from build123d import *

# Parameters (mm, degrees)
SKETCH1_W           = 31
SKETCH1_H           = 12
BOSS_EXTRUDE1_DEPTH = 11.3
SKETCH3_W           = 2
SKETCH3_H           = 4.45
BOSS_EXTRUDE2_DEPTH = 12
SKETCH4_W           = 2
SKETCH4_H           = 4.45
BOSS_EXTRUDE3_DEPTH = 12
SKETCH5_R           = 1
CUT_EXTRUDE1_DEPTH  = 36.285443174
SKETCH6_R           = 6
BOSS_EXTRUDE4_DEPTH = 3
SKETCH8_R           = 4
BOSS_EXTRUDE5_DEPTH = 3


with BuildPart() as part:
    # Sketch1 → Boss-Extrude1 (new, symmetric)
    with BuildSketch(Plane(origin=(0, 0, 0), x_dir=(1, 0, 0), z_dir=(0, 1, 0))):
        Rectangle(SKETCH1_W, SKETCH1_H)
    extrude(amount=BOSS_EXTRUDE1_DEPTH, both=True)

    # Sketch3 → Boss-Extrude2 (add)
    with BuildSketch(Plane(origin=(0, 0, -6), x_dir=(-1, 0, 0), z_dir=(0, 0, -1))):
        with Locations((14.5, 13.525)):
            Rectangle(SKETCH3_W, SKETCH3_H)
    extrude(amount=-BOSS_EXTRUDE2_DEPTH)

    # Sketch4 → Boss-Extrude3 (add)
    with BuildSketch(Plane(origin=(0, 0, -6), x_dir=(-1, 0, 0), z_dir=(0, 0, -1))):
        with Locations((14.5, -13.525)):
            Rectangle(SKETCH4_W, SKETCH4_H)
    extrude(amount=-BOSS_EXTRUDE3_DEPTH)

    # Sketch5 → Cut-Extrude1 (cut, through all)
    with BuildSketch(Plane.ZY.offset(15.5)):
        with Locations((0, 14.65)):
            Circle(SKETCH5_R)
        with Locations((0, -14.65)):
            Circle(SKETCH5_R)
    extrude(amount=-CUT_EXTRUDE1_DEPTH, mode=Mode.SUBTRACT)

    # Sketch6 → Boss-Extrude4 (add, symmetric)
    with BuildSketch(Plane.ZY.offset(15.5)):
        with Locations((0, 6.07521459)):
            Circle(SKETCH6_R)
    extrude(amount=BOSS_EXTRUDE4_DEPTH, both=True)

    # Sketch8 → Boss-Extrude5 (add, symmetric)
    with BuildSketch(Plane.ZY.offset(18.5)):
        with Locations((0, 6.07521459)):
            Circle(SKETCH8_R)
    extrude(amount=BOSS_EXTRUDE5_DEPTH, both=True)


solid = part.part
Check sheet for the modelled part. Datum: model origin and axes. Units: mm. A direction names the side the tool comes from. Round coordinates to 2 decimals unless told otherwise and drop trailing zeros. Loops run counter-clockwise (first coordinate to the right, second up) from the corner with the lowest first, then second, coordinate; pieces in that order, holes last.
1. Sectioned sample at A-A on y = 14.65. Record the boundary of the cut face in (x, z), and give its area (3 significant figures).
2. Sectioned sample at C-C on x = -13. Record the boundary of the cut face in (y, z), and give its area (3 significant figures).
3. Mould release check, pull along Z, two halves, no side actions. Record for faces 1 (the cylindrical face through (-14.51, 15.49, 0.54)), 2 (the flat face through (-18.5, 2, 1)), 3 (the cylindrical face through (-13.007, 12.075, 0.043)): released by +Z, released by -Z, zero draft, split by the parting line, or undercut.
4. Sectioned sample at D-D on y = -0.5. Record the boundary of the cut face in (x, z), and give its area (3 significant figures).
5. Scan lines: probe 1 along Y at (x, z) = (-14, -0.5); probe 2 along Y at (x, z) = (4.5, -3.75); probe 3 along X at (y, z) = (-10, -3). Record each from-to range of solid material in increasing order.
6. Gauge pin test, flat ends, axial feed: pin 1 Ø1.2 at (y, z) = (14.65, 0) entering from +X; pin 2 Ø6 at (y, z) = (-6.5, -4.5) entering from -X; pin 3 Ø2 at (y, z) = (14.5, -0.5) entering from +X; pin 4 Ø0.9 at (y, z) = (12, -1) entering from +X. Record the tip position at first contact, or that the pin passes through.
7. Set-up check for faces 4 (the cylindrical face through (-20.02, 10.04, -0.52)), 5 (the flat face through (0, 0, -6)), 6 (the cylindrical face through (-14.514, -14.35, 0.954)), 7 (the flat face through (1, -11.3, 0)), 8 (the flat face through (-15.5, 13, 0)): record each of +Z, -Z, +X, -X, +Y, -Y from which the full face is reachable in a straight line by a thin tool's end or side.
8. Sectioned sample at B-B on z = 0. Record the boundary of the cut face in (x, y), and give its area (3 significant figures).
Recorded:
1. outline: (-15.5, -6) - (-13.5, -6) - (-13.5, -1) - (-15.5, -1) - close; (-15.5, 1) - (-13.5, 1) - (-13.5, 6) - (-15.5, 6) - close
1. area: 20.0 mm2
2. outline: (-11.3, -6) - (11.3, -6) - (11.3, -2.95) arc R6 ccw to (11.3, 2.95) - (11.3, 6) - (-11.3, 6) - close
2. area: 274 mm2
3. face 1: undercut
3. face 2: zero draft
3. face 3: split by the parting line
4. outline: (-15.5, -6) - (15.5, -6) - (15.5, 6) - (-15.5, 6) - close
4. area: 372 mm2
5. probe 1: y = -15.75 to -15.52, -13.78 to 13.78, 15.52 to 15.75
5. probe 2: y = -11.3 to 11.3
5. probe 3: x = -15.5 to 15.5
6. pin 1: passes through
6. pin 2: stops at x = -15.5
6. pin 3: stops at x = -13.5
6. pin 4: stops at x = -12.5
7. face 4: -X
7. face 5: -Z, +X, -X, +Y, -Y
7. face 6: +X, -X
7. face 7: +Z, -Z, +X, -Y
7. face 8: -X, +Y
8. outline: (-21.5, 2.08) - (-18.5, 2.08) - (-18.5, 0.08) - (-15.5, 0.08) - (-15.5, -13.65) - (-13.5, -13.65) - (-13.5, -11.3) - (15.5, -11.3) - (15.5, 11.3) - (-12.5, 11.3) - (-12.5, 12.08) - (-13.5, 12.08) - (-13.5, 13.65) - (-15.5, 13.65) - (-15.5, 12.08) - (-18.5, 12.08) - (-18.5, 10.08) - (-21.5, 10.08) - close; (-15.5, -15.75) - (-13.5, -15.75) - (-13.5, -15.65) - (-15.5, -15.65) - close; (-15.5, 15.65) - (-13.5, 15.65) - (-13.5, 15.75) - (-15.5, 15.75) - close
8. area: 771 mm2
